Here's how the part is built. I have some questions about the finished solid (model axes, mm). Round coordinates to 2 decimals unless told otherwise and drop trailing zeros. Order: outer loops, then holes, each group sorted by start corner. A loop starts at its lowest first (then second) coordinate and runs counter-clockwise, first axis right, second up. Notation, with made-up numbers: (7.25, 84.25) -> (25.25, 84.25) arc R21 cw to (25.25, 100.25) -> close; hole circle Ø5 at (4, 23.25). An arc over 180 degrees is marked (long way). Use a Markdown table: item, result. Add a question column.
(1) I'm going to push flat-ended pins straight in: P1, Ø5, axis at x = 12.7, z = 0, coming from the -Y side; P2, Ø2, axis at x = 12, z = 1, coming from the +Y side; P3, Ø5, axis at x = 50.8, y = 4.76, coming from the -Z side. Where does each tip first touch, or does it pass through?
(2) Thinking about a two-plate mould opening in X: for faces 1 (the face through (63, 0, 0)), 2 (the face through (86.72, 4.7, -0.1)), 3 (the face through (-3.555, 4.701, 3.589)), which applies, pulls with the +X half, pulls with the -X half, needs draft (parallel to the pull), parting line crosses it, or undercut?
(3) I want a section at A-A, the plane x = 88.9. Please give me the cut outline in (y, z) (1 decimal).
(4) I want a section at B-B, the plane z = 0. Give the number of separate pieces and of enclosed holes in the cut face, then the cut area to 3 significant figures.
(5) If I drill on probe 1 along X at (y, z) = (1, 0.25); probe 2 along X at (y, z) = (4.75, 2.25); probe 3 along X at (y, z) = (6.25, -3), over which ranges is the centre line in solid material (lowest first)?
from build123d import *

# Parameters (mm, degrees)
SKETCH1_W               = 136.525
SKETCH1_H               = 9.525
SKETCH1_R               = 2.1828125
BOSS_EXTRUDE1_DEPTH     = 9.525
SKETCH2_R               = 2.1828125
CUT_EXTRUDE1_DEPTH      = 1
CUT_EXTRUDE1_DEPTH_BACK = 10.525
CHAMFER1_SIZE           = 2.38125
CHAMFER2_SIZE           = 0.396875


with BuildPart() as part:
    # Sketch1 → Boss-Extrude1 (new body)
    with BuildSketch(Plane(origin=(0, 0, 0), x_dir=(1, 0, 0), z_dir=(0, 1, 0))):
        with Locations((63.5, 0)):
            Rectangle(SKETCH1_W, SKETCH1_H)
        Circle(SKETCH1_R, mode=Mode.SUBTRACT)
        with Locations((12.7, 0)):
            Circle(SKETCH1_R, mode=Mode.SUBTRACT)
        with Locations((127, 0)):
            Circle(SKETCH1_R, mode=Mode.SUBTRACT)
        with Locations((88.9, 0)):
            Circle(SKETCH1_R, mode=Mode.SUBTRACT)
    extrude(amount=BOSS_EXTRUDE1_DEPTH)

    # Sketch2 → Cut-Extrude1 (cut, two sides)
    with BuildSketch(Plane.XY.offset(4.7625)) as cut_extrude1_sk:
        with Locations((25.4, 4.7625)):
            Circle(SKETCH2_R)
        with Locations((50.8, 4.7625)):
            Circle(SKETCH2_R)
    extrude(amount=CUT_EXTRUDE1_DEPTH, mode=Mode.SUBTRACT)
    extrude(cut_extrude1_sk.sketch, amount=-CUT_EXTRUDE1_DEPTH_BACK, mode=Mode.SUBTRACT)

    # Chamfer1
    chamfer1_edges = [part.edges().sort_by_distance(p)[0] for p in [
        (-4.7625, 4.7625, -4.7625),
        (131.7625, 4.7625, -4.7625),
        (131.7625, 4.7625, 4.7625),
        (-4.7625, 4.7625, 4.7625),
    ]]
    chamfer(chamfer1_edges, length=CHAMFER1_SIZE)

    # Chamfer2
    chamfer2_edges = [part.edges().sort_by_distance(p)[0] for p in [
        (-2.1828125, 0, 0),
        (-2.1828125, 9.525, 0),
        (10.5171875, 0, 0),
        (10.5171875, 9.525, 0),
        (124.8171875, 0, 0),
        (124.8171875, 9.525, 0),
        (86.7171875, 0, 0),
        (86.7171875, 9.525, 0),
        (23.2171875, 4.7625, -4.7625),
        (23.2171875, 4.7625, 4.7625),
        (48.6171875, 4.7625, -4.7625),
        (48.6171875, 4.7625, 4.7625),
        (63.5, 0, -4.7625),
        (63.5, 9.525, -4.7625),
        (-4.7625, 0, 0),
        (131.7625, 0, 0),
        (63.5, 0, 4.7625),
        (-3.571875, 0, 3.571875),
        (-3.571875, 0, -3.571875),
        (130.571875, 0, 3.571875),
        (130.571875, 0, -3.571875),
        (131.7625, 9.525, 0),
        (-4.7625, 9.525, 0),
        (63.5, 9.525, 4.7625),
        (-3.571875, 9.525, 3.571875),
        (-3.571875, 9.525, -3.571875),
        (130.571875, 9.525, 3.571875),
        (130.571875, 9.525, -3.571875),
    ]]
    chamfer(chamfer2_edges, length=CHAMFER2_SIZE)


solid = part.part
Taken from the geometry:
| question | item | result |
|---|---|---|
| 1 | P1 | stops at y = 0.08 |
| 1 | P2 | stops at y = 9.17 |
| 1 | P3 | stops at z = -4.69 |
| 2 | face 1 | needs draft |
| 2 | face 2 | undercut |
| 2 | face 3 | pulls with the -X half |
| 3 | outline | (0, -4.4) -> (0.4, -4.8) -> (9.1, -4.8) -> (9.5, -4.4) -> (9.5, -2.6) -> (9.1, -2.2) -> (0.4, -2.2) -> (0, -2.6) -> close; (0, 2.6) -> (0.4, 2.2) -> (9.1, 2.2) -> (9.5, 2.6) -> (9.5, 4.4) -> (9.1, 4.8) -> (0.4, 4.8) -> (0, 4.4) -> close |
| 4 | separate pieces | 5 |
| 4 | enclosed holes | 2 |
| 4 | area | 1,100 mm2 |
| 5 | probe 1 | x = -4.76 to -2.17, 2.17 to 10.53, 14.87 to 86.73, 91.07 to 124.83, 129.17 to 131.76 |
| 5 | probe 2 | x = -4.76 to 23.22, 27.58 to 48.62, 52.98 to 131.76 |
| 5 | probe 3 | x = -4.14 to 23.8, 27 to 49.2, 52.4 to 131.14 |
